Autodesk Inventor part; units mm, degrees
ref_plane "YZ Plane" through (0, 0, 0) normal (1, 0, 0) x (0, 1, 0)
ref_plane "XZ Plane" through (0, 0, 0) normal (0, 1, 0) x (-1, 0, 0)
ref_plane "XY Plane" through (0, 0, 0) normal (0, 0, 1) x (1, 0, 0)
sketch "Sketch1" plane through (0, 0, 0) normal (0, 0, 1) x (1, 0, 0)
  line L0 (-19.4444, 0) -> (31.3556, 0)
  line L1 (31.3556, 0) -> (31.3556, 12.7)
  line L2 (31.3556, 12.7) -> (-19.4444, 12.7)
  line L3 (-19.4444, 12.7) -> (-19.4444, 0)
  circle A0 centre (5.9556, 12.7) radius 6.35
  circle A1 centre (5.9556, 12.7) radius 12.7
  point P0 (0, 0)
  dimension "d0" = 50.8
  dimension "d2" = 12.7
  dimension "d3" = 12.7
  dimension "d4" = 25.4
extrude "Extrusion1" add sketch "Sketch1" against normal blind 25.4 contours L3 L2 A1 L0 | A1 L2 L1 L0 | A1 L2 A0 | A1 L2 A0 | L2 A0 picked at (5.205, 10.7209)
extrude "Extrusion2" cut sketch "Sketch1" against normal blind 25.4 contours A0 L2 | L2 A0
properties part number "proxybearing"
Part model, mm, in its own coordinate system. A direction names the side the tool comes from. Coordinates: 2 decimals unless noted, no trailing zeros. Order: outer loops, then holes, each group sorted by start corner. A loop starts at its lowest first (then second) coordinate and runs counter-clockwise, first axis right, second up. Notation, with made-up numbers: (-14, 31.25) - (7, 31.25) arc R25 ccw to (7, 64.25) - close; hole circle Ø5 at (5, -28.5). An arc over 180 degrees is marked (long way). Return JSON: item names as keys, results as strings. Group by question number.
Item 1: Cut at B-B (z = -17). List the corners of the cut face in (x, y).
Item 2: Cut at D-D (x = -6). List the corners of the cut face in (y, z).
Item 3: Which spindle directions (+Z, -Z, +X, -X, +Y, -Y) get a long thin tool onto all of the face, cutting with end or side? Do faces 1 (the face through (-19.444, 6, -13)), 2 (the face through (-13, 12.7, -13)). Say none if no direction does.
Item 4: Cut at A-A (y = 15.5). List the corners of the cut face in (x, z).
Item 5: Drill centre lines: probe 1 along Y at (x, z) = (6, -24); probe 2 along Y at (x, z) = (-7.5, -15.5); probe 3 along Y at (x, z) = (1, -6.5). Where is each one in solid material? Low to high. Write a range as from..to.
Item 6: Pull direction Y, two halves, no side cores. Call faces 3 (the face through (25, 12.7, -13)), 4 (the face through (5.129, 18.996, -12.522)), 5 (the face through (6, 0, -13)): pulls with the +Y half, pulls with the -Y half, needs draft (parallel to the pull), parting line crosses it, or undercut.
Item 7: Pin check, flat tips, straight feed: pin 1 (2 mm diameter, centred on x = 14.5, z = -16.5, fed in from +Y); pin 2 (10 mm diameter, centred on x = 24.5, z = -12.5, fed in from +Y); pin 3 (1 mm diameter, centred on x = 13, z = -4, fed in from +Y). Stop position of each tip, or through.
Item 8: Cut at C-C (y = 8.5). List the corners of the cut face in (x, z).
Check values:
{
 "1": {"outline": "(-19.44, 0) - (31.36, 0) - (31.36, 12.7) - (18.66, 12.7) arc R12.7 ccw to (-6.74, 12.7) - (-19.44, 12.7) - close; hole circle Ø12.7 at (5.96, 12.7)"},
 "2": {"outline": "(0, -25.4) - (16.98, -25.4) - (16.98, 0) - (0, 0) - close"},
 "3": {"face 1": "+Z, -Z, -X, +Y, -Y", "face 2": "+Z, -Z, -X, +Y"},
 "4": {"outline": "(-6.43, -25.4) - (0.26, -25.4) - (0.26, 0) - (-6.43, 0) - close; (11.65, -25.4) - (18.34, -25.4) - (18.34, 0) - (11.65, 0) - close"},
 "5": {"probe 1": "y = 0..6.35, 19.05..25.4", "probe 2": "y = 0..12.7", "probe 3": "y = 0..8.73, 16.67..24.39"},
 "6": {"face 3": "pulls with the +Y half", "face 4": "undercut", "face 5": "pulls with the -Y half"},
 "7": {"pin 1": "stops at y = 22.92", "pin 2": "stops at y = 12.7", "pin 3": "stops at y = 23.58"},
 "8": {"outline": "(-19.44, -25.4) - (1.19, -25.4) - (1.19, 0) - (-19.44, 0) - close; (10.72, -25.4) - (31.36, -25.4) - (31.36, 0) - (10.72, 0) - close"}
}
